```python
from build123d import *

# Parameters (mm, degrees)
SKETCH1_R           = 1.5875
BOSS_EXTRUDE1_DEPTH = 9.525


with BuildPart() as part:
    # Sketch1 → Boss-Extrude1 (new body)
    with BuildSketch(Plane(origin=(0, 0, 0), x_dir=(0, 0, -1), z_dir=(1, 0, 0))):
        Polygon((0, 1.5875), (0, -1.5875), (-17.78, -1.5875), (-17.78, -4.7625), (-30.48, -4.7625), (-30.48, -1.5875), (-53.975, -1.5875), (-53.975, -4.7625), (-57.15, -4.7625), (-57.15, 1.5875), align=None)
        with Locations((-24.13, -1.5875)):
            Circle(SKETCH1_R, mode=Mode.SUBTRACT)
    extrude(amount=BOSS_EXTRUDE1_DEPTH)


solid = part.part
```
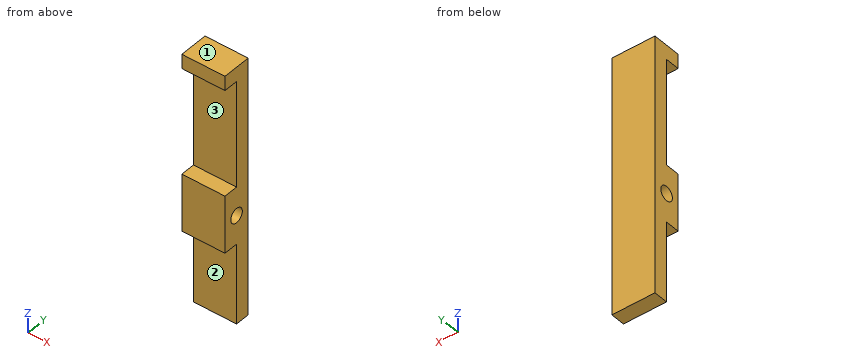
Input: part model. Units: mm. Frame: model coordinates. Face numbers are marked on the shaded views. A direction names the side the tool comes from. Round coordinates to 2 decimals unless told otherwise and drop trailing zeros. Loops run counter-clockwise (first coordinate to the right, second up) from the corner with the lowest first, then second, coordinate; pieces in that order, holes last.
1) Set-up query: the marked faces 1, 2 and 3. Return all of +Z, -Z, +X, -X, +Y, -Y with unobstructed straight access to the full face (end or side cutting, diameter ignored); none if empty.
Ans:
face 1: +Z, +X, -X, +Y, -Y
face 2: -Z, +X, -X, -Y
face 3: +X, -X, -Y
2) Section query A-A on z = 24.13. Return the cut outline in (x, y) (1 decimal).
Ans:
outline: (0, -4.8) - (9.5, -4.8) - (9.5, -3.2) - (0, -3.2) - close; (0, 0) - (9.5, 0) - (9.5, 1.6) - (0, 1.6) - close
3) Section query D-D on z = 9. Return the cut outline in (x, y) (1 decimal).
Ans:
outline: (0, -1.6) - (9.5, -1.6) - (9.5, 1.6) - (0, 1.6) - close
4) Material intervals for line 1 (Y direction, x = 6.25, z = 24.13) (1 decimal); line 2 (Z direction, x = 1, y = -1.5); line 3 (Z direction, x = 2.5, y = -2.5) (3 decimals), sorted ascending.
Ans:
line 1: y = -4.8 to -3.2, 0 to 1.6
line 2: z = 0 to 22.54, 25.72 to 57.15
line 3: z = 17.78 to 22.831, 25.429 to 30.48, 53.975 to 57.15
5) Pin query (flat end, axial travel): pin 1 (2 mm diameter, centred on y = -3, z = 17.5, fed in from +X) (3 decimals); pin 2 (1 mm diameter, centred on x = 5.5, y = -3, fed in from -Z); pin 3 (5 mm diameter, centred on x = 5, z = 4.5, fed in from -Y); pin 4 (3 mm diameter, centred on y = -1.59, z = 24.13, fed in from -X). Return the tip coordinate at first contact, or that it passes through.
Ans:
pin 1: stops at x = 9.525
pin 2: stops at z = 17.78
pin 3: stops at y = -1.59
pin 4: passes through
6) Section query C-C on y = -3.75. Return the cut outline in (x, z) (3 decimals), plus the area to 3 significant figures.
Ans:
outline: (0, 17.78) - (9.525, 17.78) - (9.525, 30.48) - (0, 30.48) - close; (0, 53.975) - (9.525, 53.975) - (9.525, 57.15) - (0, 57.15) - close
area: 151 mm2
